The drawing under review shows one solid part. Ordinate dimensions are in mm from its lowest x, y, z. Coordinates: 2 decimals unless noted, no trailing zeros. Write each loop counter-clockwise with the first axis right and the second up, starting at its lowest first coordinate (ties: lowest second). Pieces come first, ordered by that corner, then holes. Notation, with made-up numbers: M -11,-39.75 L 46,-39.75 A15 cw 46,-11.75 Z; hole C 5,-1.5 d9. An arc over 180 degrees is marked long. Write each question's results on one line, items separated by ' | '. Start each with the question number.
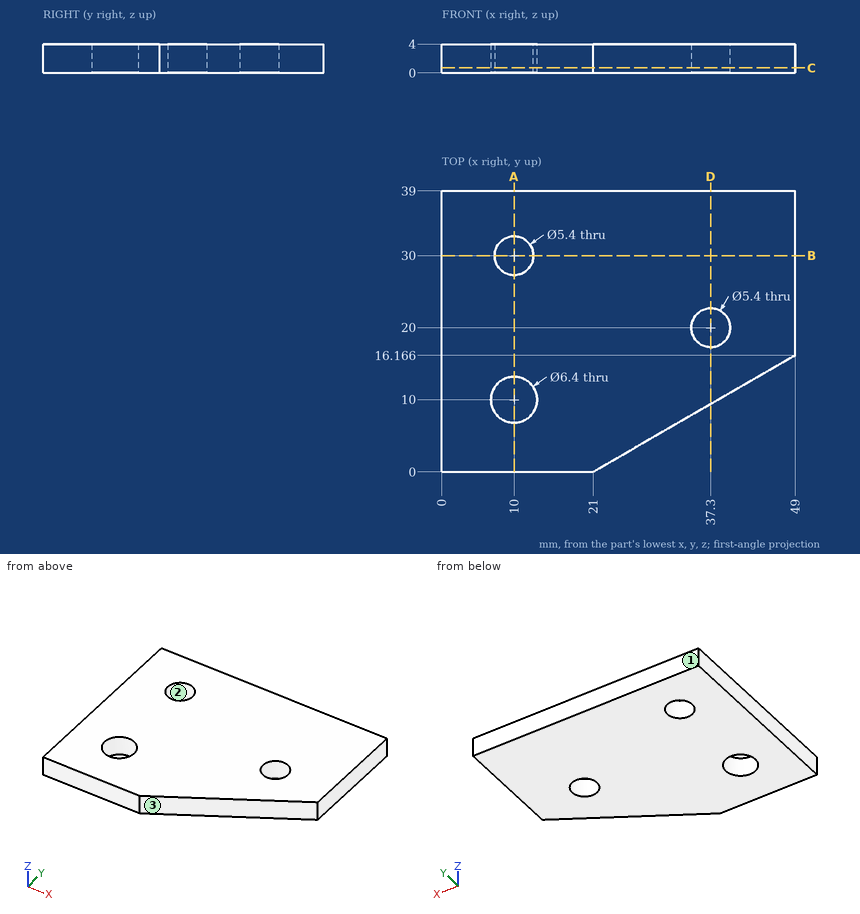
Item 1: We need section A-A on x = 10. State the section outline as (y, z) points.
Item 2: We need section B-B on y = 30. State the section outline as (x, z) points.
Item 3: Draft analysis for pull direction Y (two halves, no side actions). For the marked faces 1, 2 and 3, state which applies: released by +Y, released by -Y, zero draft, split by the parting line, or undercut.
Item 4: We need section C-C on z = 0.7. State the section outline as (x, y) points.
Item 5: We need section D-D on x = 37.3. State the section outline as (y, z) points.
Item 6: Wall thickness on L1, parallel to Y at x = 10, z = 1.5; L2, parallel to X at y = 20, z = 0.2; L3, parallel to X at y = 30, z = 1.35: over which ranges is each line inside the solid? List them lowest first.
Answer:
1) outline: M 0,0 L 6.8,0 L 6.8,4 L 0,4 Z; M 13.2,0 L 27.3,0 L 27.3,4 L 13.2,4 Z; M 32.7,0 L 39,0 L 39,4 L 32.7,4 Z
2) outline: M 0,0 L 7.3,0 L 7.3,4 L 0,4 Z; M 12.7,0 L 49,0 L 49,4 L 12.7,4 Z
3) face 1: released by +Y | face 2: undercut | face 3: released by -Y
4) outline: M 0,0 L 21,0 L 49,16.17 L 49,39 L 0,39 Z; hole C 10,10 d6.4; hole C 10,30 d5.4; hole C 37.3,20 d5.4
5) outline: M 9.41,0 L 17.3,0 L 17.3,4 L 9.41,4 Z; M 22.7,0 L 39,0 L 39,4 L 22.7,4 Z
6) L1: y = 0 to 6.8, 13.2 to 27.3, 32.7 to 39 | L2: x = 0 to 34.6, 40 to 49 | L3: x = 0 to 7.3, 12.7 to 49
